```python
from build123d import *

# Parameters (mm, degrees)
BOSS_EXTRUDE1_DEPTH          = 0.635
F_97_0_0059_DIAMETER_HOLE1_D = 2.921
CUT_EXTRUDE8_DEPTH           = 0.635


with BuildPart() as part:
    # Sketch1 → Boss-Extrude1 (new, symmetric)
    with BuildSketch(Plane(origin=(0, 0, 0), x_dir=(1, 0, 0), z_dir=(0, 1, 0))):
        Polygon((-41.424046485, -10.283259465), (-41.424046485, -12.505759465), (-47.774046485, -12.505759465), (-47.774046485, -6.155759465), (-41.424046485, -6.155759465), (-41.424046485, -8.378259465), (-9.674046485, -8.378259465), (-9.674046485, -6.155759465), (-3.324046485, -6.155759465), (-3.324046485, -12.505759465), (-9.674046485, -12.505759465), (-9.674046485, -10.283259465), align=None)
    extrude(amount=BOSS_EXTRUDE1_DEPTH, both=True)

    # #97 (0.0059) Diameter Hole1 (through all)
    with Locations(Plane(origin=(0, 0.635, 0), x_dir=(-1, 0, 0), z_dir=(0, 1, 0))):
        with Locations((44.599046485, 9.330759465)):
            f_97_0_0059_diameter_hole1 = Hole(F_97_0_0059_DIAMETER_HOLE1_D / 2)

    # Mirror1: #97 (0.0059) Diameter Hole1 across plane
    add(f_97_0_0059_diameter_hole1.mirror(Plane(origin=(-25.549046485, 0, 0), x_dir=(0, 0, 1), z_dir=(1, 0, 0))), mode=Mode.SUBTRACT)

    # Sketch5 → Cut-Extrude8 (cut)
    with BuildSketch(Plane(origin=(0, 0.635, 0), x_dir=(1, 0, 0), z_dir=(0, 1, 0))):
        with BuildLine():
            Line((-15.39166679, -8.378259465), (-35.821920417, -8.378259465))
            ThreePointArc((-35.821920417, -8.378259465), (-36.774420417, -9.330759465), (-35.821920417, -10.283259465))
            Line((-35.821920417, -10.283259465), (-15.39166679, -10.283259465))
            ThreePointArc((-15.39166679, -10.283259465), (-14.43916679, -9.330759465), (-15.39166679, -8.378259465))
        make_face()
    extrude(amount=-CUT_EXTRUDE8_DEPTH, mode=Mode.SUBTRACT)


solid = part.part
```
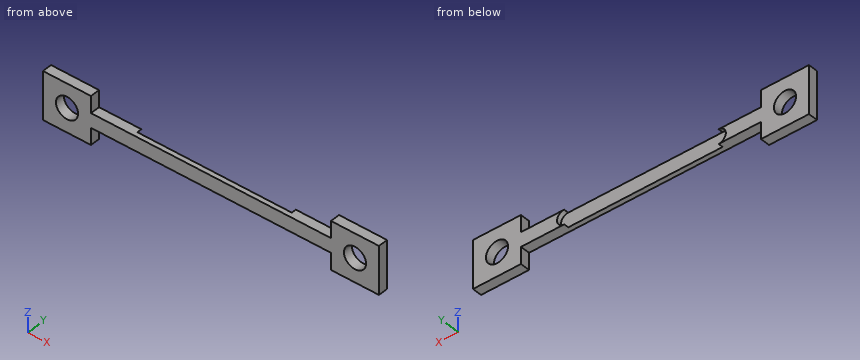
Model file for the job. Use its own axes, mm. Coordinates: 2 decimals unless noted, no trailing zeros. Order: outer loops, then holes, each group sorted by start corner. A loop starts at its lowest first (then second) coordinate and runs counter-clockwise, first axis right, second up. Notation, with made-up numbers: (-6.75, 75) -> (46.25, 75) arc R3 ccw to (46.25, 80) -> close; hole circle Ø9 at (-9, -7.5). An arc over 180 degrees is marked (long way). Answer as a JSON object with one key per item and string values. Group by question number.
1) Cut at A-A, the plane y = 0.25. Write the cut outline in (x, z) (1 decimal), then the cut area to 3 significant figures.
2) Cut at D-D, the plane x = -11. Write the cut outline in (y, z) (3 decimals), then the cut area to 3 significant figures.
3) Flat gauge pin, fed straight in: pin 1 (0.6 mm diameter, centred on x = -26.5, z = 9, fed in from +Y). Where does the tip first touch, or does it go through?
4) Cut at B-B, the plane z = 8.75. Write the cut outline in (x, y) (3 decimals).
5) Cut at C-C, the plane x = -26. Write the cut outline in (y, z) (3 decimals), then the cut area to 3 significant figures.
6) Drill centre lines: L1, parallel to X at y = 0, z = 6.5; L2, parallel to X at y = 0.5, z = 9.25; L3, parallel to X at y = 0, z = 10.5. Where is each one in solid material? Low to high.
Check values:
{
 "1": {"outline": "(-47.8, 6.2) -> (-41.4, 6.2) -> (-41.4, 8.4) -> (-35.8, 8.4) arc R1 cw to (-35.8, 10.3) -> (-41.4, 10.3) -> (-41.4, 12.5) -> (-47.8, 12.5) -> close; (-15.4, 8.4) -> (-9.7, 8.4) -> (-9.7, 6.2) -> (-3.3, 6.2) -> (-3.3, 12.5) -> (-9.7, 12.5) -> (-9.7, 10.3) -> (-15.4, 10.3) arc R1 cw to start; hole circle Ø2.9 at (-44.6, 9.3); hole circle Ø2.9 at (-6.5, 9.3)", "area": "86.0 mm²"},
 "2": {"outline": "(-0.635, 8.378) -> (0.635, 8.378) -> (0.635, 10.283) -> (-0.635, 10.283) -> close", "area": "2.42 mm²"},
 "3": {"pin 1": "stops at y = 0"},
 "4": {"outline": "(-47.774, -0.635) -> (-45.939, -0.635) -> (-45.939, 0.635) -> (-47.774, 0.635) -> close; (-43.259, -0.635) -> (-7.839, -0.635) -> (-7.839, 0.635) -> (-14.637, 0.635) -> (-14.637, 0) -> (-36.577, 0) -> (-36.577, 0.635) -> (-43.259, 0.635) -> close; (-5.159, -0.635) -> (-3.324, -0.635) -> (-3.324, 0.635) -> (-5.159, 0.635) -> close"},
 "5": {"outline": "(-0.635, 8.378) -> (0, 8.378) -> (0, 10.283) -> (-0.635, 10.283) -> close", "area": "1.21 mm²"},
 "6": {"L1": "x = -47.77 to -41.42, -9.67 to -3.32", "L2": "x = -47.77 to -46.06, -43.14 to -36.77, -14.44 to -7.96, -5.04 to -3.32", "L3": "x = -47.77 to -45.47, -43.72 to -41.42, -9.67 to -7.37, -5.62 to -3.32"}
}
